Input: part model. Units: mm. Frame: model coordinates. A direction names the side the tool comes from. Coordinates: 2 decimals unless noted, no trailing zeros. Write each loop counter-clockwise with the first axis right and the second up, starting at its lowest first coordinate (ties: lowest second). Pieces come first, ordered by that corner, then holes. Notation, with made-up numbers: (11.25, 0) - (28.25, 0) arc R15 cw to (28.25, 18) - close; hole circle Ø2 at (51.25, -24.5). An arc over 180 degrees is marked (long way). Use CSV: the item, a comma, the result in double quotes.
```python
from build123d import *

# Parameters (mm, degrees)
F0_W     = 50
F0_H     = 200
F0_W_2   = 40
F0_H_2   = 190
F1_DEPTH = 50
F2_R     = 15
F3_DEPTH = 5


with BuildPart() as f1:
    # F0 (on Front) → F1 (new body)
    with BuildSketch(Plane.XZ):
        with Locations((25, 100)):
            Rectangle(F0_W, F0_H)
        with Locations((25, 100)):
            Rectangle(F0_W_2, F0_H_2, mode=Mode.SUBTRACT)
    extrude(amount=F1_DEPTH)

    # F2 (on face) → F3 (cut, through all)
    with BuildSketch(Plane.XY.offset(200)):
        with Locations((25, -25)):
            Circle(F2_R)
    extrude(amount=-F3_DEPTH, mode=Mode.SUBTRACT)


solid = f1.part
```
(1) Cut plane C-C on y = -5. Return loops of the section in (x, z), and give its area (3 significant figures).
Check values:
outline,"(0, 0) - (50, 0) - (50, 200) - (0, 200) - close; hole (5, 5) - (45, 5) - (45, 195) - (5, 195) - close"
area,"2,400 mm^2"
(2) Draft query along Z for faces 4 (the flat face through (45, -25, 99)), 5 (the flat face through (36, -36, 200)), 6 (the flat face through (4.5, 0, 107.9)). Return one class per face: pulls with the +Z half, pulls with the -Z half, needs draft (parallel to the pull), parting line crosses it, or undercut.
Check values:
face 4,"undercut"
face 5,"pulls with the +Z half"
face 6,"needs draft"
(3) Ray query, probe 1 along Z at (x, y) = (8, -43); probe 2 along X at (y, z) = (-8.5, 33.5); probe 3 along Y at (x, z) = (25, 197). Return the intervals inside material, ascending. Write a range as from..to.
Check values:
probe 1,"0..5, 195..200"
probe 2,"0..5, 45..50"
probe 3,"-50..-40, -10..0"
(4) Pin query (flat end, axial travel): pin 1 Ø18 at (x, y) = (25, -25) entering from +Z; pin 2 Ø12 at (x, z) = (36, 56) entering from +Y. Return the tip coordinate at first contact, or that it passes through.
Check values:
pin 1,"z = 5"
pin 2,"through"
(5) Reachability of faces 1 (the flat face through (25, -41, 195)), 2 (the cylindrical face through (21.748, -39.643, 197.535)), 3 (the flat face through (0, -25, 99)) from +Z, -Z, +X, -X, +Y, -Y: full face, straight path, thin tool, end or side. Return the list, or none.
Check values:
face 1,"+Y, -Y"
face 2,"+Z"
face 3,"+Z, -Z, -X, +Y, -Y"
(6) Cut plane B-B on x = 25. Return loops of the section in (y, z).
Check values:
outline,"(-50, 0) - (0, 0) - (0, 5) - (-50, 5) - close; (-50, 195) - (-40, 195) - (-40, 200) - (-50, 200) - close; (-10, 195) - (0, 195) - (0, 200) - (-10, 200) - close"
(7) Cut plane A-A on z = 53.5. Return loops of the section in (x, y).
Check values:
outline,"(0, -50) - (5, -50) - (5, 0) - (0, 0) - close; (45, -50) - (50, -50) - (50, 0) - (45, 0) - close"
(8) Cut plane D-D on y = -25. Return loops of the section in (x, z).
Check values:
outline,"(0, 0) - (50, 0) - (50, 200) - (40, 200) - (40, 195) - (45, 195) - (45, 5) - (5, 5) - (5, 195) - (10, 195) - (10, 200) - (0, 200) - close"
